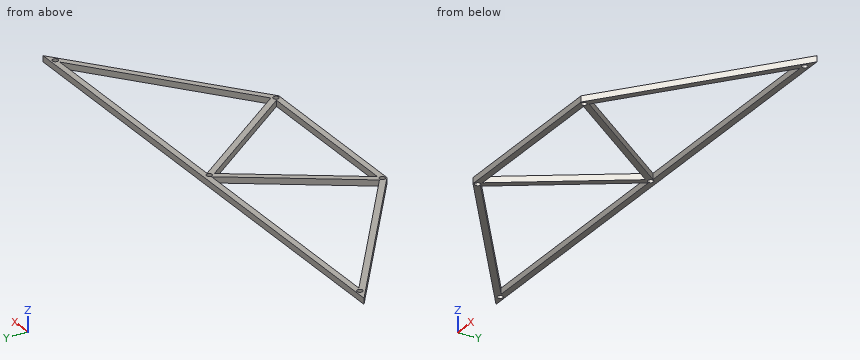
```python
from build123d import *

# Parameters (mm, degrees)
BOSS_EXTRUDE1_DEPTH = 15
SKETCH2_R           = 7
CUT_EXTRUDE2_DEPTH  = 15


with BuildPart() as part:
    # Sketch1 → Boss-Extrude1 (new body)
    with BuildSketch(Plane.XY):
        Polygon((-644.492210058, 15), (643.375012356, 15), (223.310378922, -315), (-210.705614848, -315), align=None)
        Polygon((9.272865978, 0), (600, 0), (224.024883315, -295.363567011), align=None, mode=Mode.SUBTRACT)
        Polygon((-9.092968645, 0), (-600, 0), (-211.624925428, -295.453515678), align=None, mode=Mode.SUBTRACT)
        Polygon((208.850194536, -300), (-196.555581164, -300), (0.180367696, -13.001697737), align=None, mode=Mode.SUBTRACT)
    extrude(amount=BOSS_EXTRUDE1_DEPTH)

    # Sketch2 → Cut-Extrude2 (cut)
    with BuildSketch(Plane.XY.offset(15)):
        with Locations((-611.831081684, 4.904990628)):
            Circle(SKETCH2_R)
        Circle(SKETCH2_R)
        with Locations((611.879096148, 3.706278654)):
            Circle(SKETCH2_R)
        with Locations((-207.544546049, -305.21160756)):
            Circle(SKETCH2_R)
        with Locations((219.201774513, -305.21160756)):
            Circle(SKETCH2_R)
    extrude(amount=-CUT_EXTRUDE2_DEPTH, mode=Mode.SUBTRACT)


solid = part.part
```
Work out the finished part from the listing and answer in its coordinate system (mm). Give positions to 0.01 mm unless a question says otherwise; leave off trailing zeros. Write each loop counter-clockwise with the first axis right and the second up, starting at its lowest first coordinate (ties: lowest second). Pieces come first, ordered by that corner, then holes. Notation, with made-up numbers: (-21, 50.25) -> (-15, 50.25) arc R12 ccw to (-15, 64.25) -> close; hole circle Ø9 at (61, 83.5). An arc over 180 degrees is marked (long way). Write each question's results on one line, items separated by ' | '.
1. Find section C-C on z = 2.75. Give the number of separate pieces and of enclosed holes in the cut face, and give its area (3 significant figures).
Data:
separate pieces: 1 | enclosed holes: 8 | area: 50,600 mm^2
2. Find section D-D on x = 337. Determine the outline of the cut face in (y, z).
Data:
outline: (-225.69, 0) -> (-206.61, 0) -> (-206.61, 15) -> (-225.69, 15) -> close; (0, 0) -> (15, 0) -> (15, 15) -> (0, 15) -> close
3. Find section B-B on x = 168. Determine the outline of the cut face in (y, z).
Data:
outline: (-315, 0) -> (-300, 0) -> (-300, 15) -> (-315, 15) -> close; (-243.82, 0) -> (-218.31, 0) -> (-218.31, 15) -> (-243.82, 15) -> close; (0, 0) -> (15, 0) -> (15, 15) -> (0, 15) -> close
4. Straight lines are drawn through the part: L1, parallel to Y at x = -144.5, z = 3; L2, parallel to X at y = -165.5, z = 1; L3, parallel to X at y = -99, z = 2. For each, find the intervals that lie inside material, in ascending order.
Data:
L1: -315 to -300, -224.06 to -197.53, 0 to 15 | L2: -407.22 to -382.45, -122.54 to -104.36, 111.06 to 129.6, 389.33 to 413.61 | L3: -494.64 to -469.86, -76.96 to -58.77, 62.71 to 81.25, 473.98 to 498.26
5. Each of these flat-tipped pins is pushed along its axis until it touches: pin 1 Ø22.5 at (x, y) = (0, 0) entering from -Z; pin 2 Ø8 at (y, z) = (-147.5, 6.5) entering from -X; pin 3 Ø3 at (y, z) = (-164.5, 12) entering from +X; pin 4 Ø4.5 at (x, z) = (-278.5, 7.5) entering from -Y. Where does it stop, or does it pass through?
Data:
pin 1: z = 0 | pin 2: x = -436.14 | pin 3: x = 416.79 | pin 4: y = -265.14
6. Find section A-A on y = -282. Determine the outline of the cut face in (x, z), and give its area (3 significant figures).
Data:
outline: (-254.08, 0) -> (-229.31, 0) -> (-229.31, 15) -> (-254.08, 15) -> close; (-202.4, 0) -> (-184.22, 0) -> (-184.22, 15) -> (-202.4, 15) -> close; (195.76, 0) -> (214.31, 0) -> (214.31, 15) -> (195.76, 15) -> close; (241.04, 0) -> (265.32, 0) -> (265.32, 15) -> (241.04, 15) -> close | area: 1,290 mm^2
